```python
from build123d import *

# Parameters (mm, degrees)
SKETCH2_R           = 1.375
BOSS_EXTRUDE1_DEPTH = 3


with BuildPart() as part:
    # Sketch2 → Boss-Extrude1 (new body)
    with BuildSketch(Plane(origin=(0, 0, 0), x_dir=(1, 0, 0), z_dir=(0, 1, 0))):
        with BuildLine():
            Line((-27, -2.75), (-17.987773433, -15.509030166))
            ThreePointArc((-17.987773433, -15.509030166), (-13.21593597, -17.100698117), (-15.25, -12.5))
            Line((-15.25, -12.5), (-23.5, 0))
            Line((-23.5, 0), (-15.25, 12.5))
            ThreePointArc((-15.25, 12.5), (-13.21593597, 17.100698117), (-17.987773433, 15.509030166))
            Line((-17.987773433, 15.509030166), (-27, 2.75))
            ThreePointArc((-27, 2.75), (-29.75, 0), (-27, -2.75))
        make_face()
        with Locations(Location((-27, 0, 0), (0, 0, 270))):
            Circle(SKETCH2_R, mode=Mode.SUBTRACT)
        with Locations(Location((-15.25, 15.25, 0), (0, 0, 270))):
            Circle(SKETCH2_R, mode=Mode.SUBTRACT)
        with Locations(Location((-15.25, -15.25, 0), (0, 0, 270))):
            Circle(SKETCH2_R, mode=Mode.SUBTRACT)
    extrude(amount=BOSS_EXTRUDE1_DEPTH)


solid = part.part
```
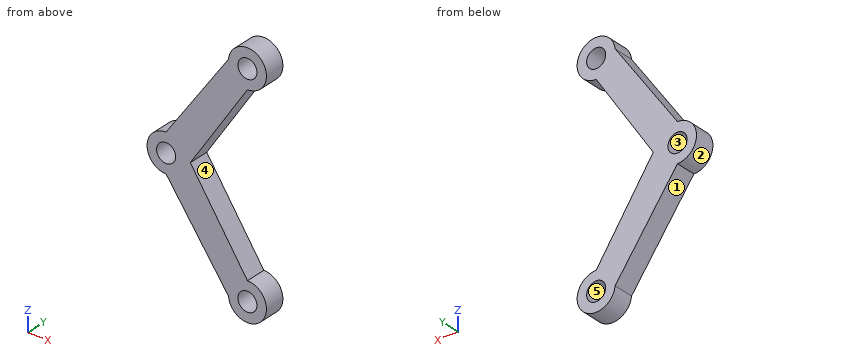
Could you check a few things on this model? Use its own coordinates, in mm. Face numbers are marked on the shaded views. A direction names the side the tool comes from. Give positions to 0.01 mm unless a question says otherwise; leave off trailing zeros. Loops run counter-clockwise (first coordinate to the right, second up) from the corner with the lowest first, then second, coordinate; pieces in that order, holes last. Notation, with made-up numbers: (-37, -15.5) -> (-11, -15.5) arc R11 ccw to (-11, 4.5) -> close; hole circle Ø6 at (27, -20). An arc over 180 degrees is marked (long way). Put each result on its own line as item: value.
(1) For the marked faces 4 and 5, which set-ups out of +Z, -Z, +X, -X, +Y, -Y let a thin tool reach every point of the face, with its end or its side?
Computed:
face 4: +X, +Y, -Y
face 5: +Y, -Y
(2) Imagine slicing it at D-D on z = -5. Write out the boundary of the cut face in (x, y).
Computed:
outline: (-25.41, 0) -> (-20.2, 0) -> (-20.2, 3) -> (-25.41, 3) -> close
(3) Imagine slicing it at B-B on z = -0.5. Write out the boundary of the cut face in (x, y), plus the area to 3 significant figures.
Computed:
outline: (-29.7, 0) -> (-28.28, 0) -> (-28.28, 3) -> (-29.7, 3) -> close; (-25.72, 0) -> (-23.17, 0) -> (-23.17, 3) -> (-25.72, 3) -> close
area: 11.9 mm^2
(4) Thinking about a two-plate mould opening in Z: for the marked faces 1, 2 and 3, which applies, pulls with the +Z half, pulls with the -Z half, needs draft (parallel to the pull), parting line crosses it, or undercut?
Computed:
face 1: pulls with the -Z half
face 2: parting line crosses it
face 3: undercut
(5) Please list where these lines run through material, in increasing order: probe 1 along Z at (x, y) = (-22.75, 2.05); probe 2 along Z at (x, y) = (-23.25, 0.35); probe 3 along X at (y, z) = (1.5, -15.25) (3 decimals). Write a range as [from, to].
Computed:
probe 1: [-8.77, -1.14], [1.14, 8.77]
probe 2: [-8.06, -0.38], [0.38, 8.06]
probe 3: [-18.171, -16.625], [-13.875, -12.5]
(6) Imagine slicing it at A-A on y = 2.55. Write out the boundary of the cut face in (x, z) (3 decimals), plus the area to 3 significant figures.
Computed:
outline: (-27, -2.75) -> (-17.988, -15.509) arc R2.75 ccw (long way) to (-15.25, -12.5) -> (-23.5, 0) -> (-15.25, 12.5) arc R2.75 ccw (long way) to (-17.988, 15.509) -> (-27, 2.75) arc R2.75 ccw to start; hole circle Ø2.75 at (-27, 0); hole circle Ø2.75 at (-15.25, -15.25); hole circle Ø2.75 at (-15.25, 15.25)
area: 175 mm^2
(7) I'm going to push flat-ended pins straight in: pin 1 Ø2.5 at (x, z) = (-15.25, -15.25) entering from +Y; pin 2 Ø1 at (y, z) = (1.5, 12.5) entering from -X. Where does each tip first touch, or does it pass through?
Computed:
pin 1: through
pin 2: x = -20.47
(8) Imagine slicing it at C-C on x = -21. Write out the boundary of the cut face in (y, z).
Computed:
outline: (0, -11.24) -> (3, -11.24) -> (3, -3.79) -> (0, -3.79) -> close; (0, 3.79) -> (3, 3.79) -> (3, 11.24) -> (0, 11.24) -> close
